Verification items for the finished model (mm, model axes). A direction names the side the tool comes from. Give positions to 0.01 mm unless a question says otherwise; leave off trailing zeros. Order: outer loops, then holes, each group sorted by start corner. A loop starts at its lowest first (then second) coordinate and runs counter-clockwise, first axis right, second up.
from build123d import *

# Parameters (mm, degrees)
BOSS_EXTRUDE2_DEPTH = 22
SHELL1_START        = -22
SHELL1_DEPTH        = 20
SKETCH2_W           = 99.356893422
SKETCH2_H           = 33.700277524
CUT_EXTRUDE1_DEPTH  = 20
SKETCH3_W           = 10.526500884
SKETCH3_H           = 10.645693642
CUT_EXTRUDE2_DEPTH  = 2
CUT_EXTRUDE3_DEPTH  = 2


# Read off the part's stored shape, not the designer's step: Shell1
with BuildPart() as part:
    # Sketch1 → Boss-Extrude2 (new body)
    with BuildSketch(Plane(origin=(0, 0, 0), x_dir=(1, 0, 0), z_dir=(0, 1, 0))):
        with BuildLine():
            Line((-51, 24.05), (51, 24.05))
            ThreePointArc((51, 24.05), (53.121320344, 23.171320344), (54, 21.05))
            Line((54, 21.05), (54, -16.2))
            ThreePointArc((54, -16.2), (53.121320344, -18.321320344), (51, -19.2))
            Line((51, -19.2), (-51, -19.2))
            ThreePointArc((-51, -19.2), (-53.121320344, -18.321320344), (-54, -16.2))
            Line((-54, -16.2), (-54, 21.05))
            ThreePointArc((-54, 21.05), (-53.121320344, 23.171320344), (-51, 24.05))
        make_face()
        with BuildLine():
            Line((-34.075, 9.25), (34.075, 9.25))
            ThreePointArc((34.075, 9.25), (43.325, 0), (34.075, -9.25))
            Line((34.075, -9.25), (-34.075, -9.25))
            ThreePointArc((-34.075, -9.25), (-43.325, 0), (-34.075, 9.25))
        make_face(mode=Mode.SUBTRACT)
    extrude(amount=-BOSS_EXTRUDE2_DEPTH)

    # Shell1 outline → Shell1 (cut)
    with BuildSketch(Plane(origin=(0, 0, 0), x_dir=(1, 0, 0), z_dir=(0, 1, 0)).offset(SHELL1_START)):
        with BuildLine():
            Line((-52, 21.05), (-52, -16.2))
            ThreePointArc((-52, -16.2), (-51.707106781, -16.907106781), (-51, -17.2))
            Line((-51, -17.2), (51, -17.2))
            ThreePointArc((51, -17.2), (51.707106781, -16.907106781), (52, -16.2))
            Line((52, -16.2), (52, 21.05))
            ThreePointArc((52, 21.05), (51.707106781, 21.757106781), (51, 22.05))
            Line((51, 22.05), (-51, 22.05))
            ThreePointArc((-51, 22.05), (-51.707106781, 21.757106781), (-52, 21.05))
        make_face()
        with BuildLine():
            ThreePointArc((-34.075, -11.25), (-45.325, 0), (-34.075, 11.25))
            Line((-34.075, 11.25), (34.075, 11.25))
            ThreePointArc((34.075, 11.25), (45.325, 0), (34.075, -11.25))
            Line((34.075, -11.25), (-34.075, -11.25))
        make_face(mode=Mode.SUBTRACT)
    extrude(amount=SHELL1_DEPTH, mode=Mode.SUBTRACT)

    # Sketch2 → Cut-Extrude1 (cut)
    with BuildSketch(Plane.XZ.offset(22)):
        Rectangle(SKETCH2_W, SKETCH2_H)
    extrude(amount=-CUT_EXTRUDE1_DEPTH, mode=Mode.SUBTRACT)

    # Sketch3 → Cut-Extrude2 (cut)
    with BuildSketch(Plane(origin=(0, 0, -24.05), x_dir=(-1, 0, 0), z_dir=(0, 0, -1))):
        with Locations((-43.321442995, -16.677153179)):
            Rectangle(SKETCH3_W, SKETCH3_H)
    extrude(amount=-CUT_EXTRUDE2_DEPTH, mode=Mode.SUBTRACT)

    # Sketch6 → Cut-Extrude3 (cut)
    with BuildSketch(Plane(origin=(0, 0, -24.05), x_dir=(-1, 0, 0), z_dir=(0, 0, -1))):
        with BuildLine():
            Line((46.497989358, -4.136848822), (-46.502010642, -4.136848822))
            ThreePointArc((-46.502010642, -4.136848822), (-47.502010642, -3.136848822), (-46.502010642, -2.136848822))
            Line((-46.502010642, -2.136848822), (46.497989358, -2.136848822))
            ThreePointArc((46.497989358, -2.136848822), (47.497989358, -3.136848822), (46.497989358, -4.136848822))
        make_face()
        with BuildLine():
            Line((46.497989358, -8.136848822), (-46.502010642, -8.136848822))
            ThreePointArc((-46.502010642, -8.136848822), (-47.502010642, -7.136848822), (-46.502010642, -6.136848822))
            Line((-46.502010642, -6.136848822), (46.497989358, -6.136848822))
            ThreePointArc((46.497989358, -6.136848822), (47.497989358, -7.136848822), (46.497989358, -8.136848822))
        make_face()
        with BuildLine():
            Line((-32.921100396, -9.626506099), (46.497989358, -9.626506099))
            ThreePointArc((46.497989358, -9.626506099), (47.497989358, -10.626506099), (46.497989358, -11.626506099))
            Line((46.497989358, -11.626506099), (-32.921100396, -11.626506099))
            ThreePointArc((-32.921100396, -11.626506099), (-33.921100396, -10.626506099), (-32.921100396, -9.626506099))
        make_face()
        with BuildLine():
            Line((-32.921100396, -13.626506099), (46.497989358, -13.626506099))
            ThreePointArc((46.497989358, -13.626506099), (47.497989358, -14.626506099), (46.497989358, -15.626506099))
            Line((46.497989358, -15.626506099), (-32.921100396, -15.626506099))
            ThreePointArc((-32.921100396, -15.626506099), (-33.921100396, -14.626506099), (-32.921100396, -13.626506099))
        make_face()
    extrude(amount=-CUT_EXTRUDE3_DEPTH, mode=Mode.SUBTRACT)


solid = part.part
(1) Go/stop test with flat-tipped pins: pin 1 (1.6 mm diameter, centred on y = -17, z = -23.5, fed in from -X); pin 2 (1 mm diameter, centred on y = -14.5, z = -23, fed in from +X); pin 3 (12 mm diameter, centred on x = 22, z = -11, fed in from -Y). Record where each tip stops, or that it passes through.
Solved:
pin 1: stops at x = -53.51
pin 2: stops at x = 53.63
pin 3: stops at y = -2
(2) Section check D-D, the plane z = -20. Enter the section's corners in (x, y), then the cut area to 3 significant figures.
Solved:
outline: (-54, -22) - (-52, -22) - (-52, -2) - (52, -2) - (52, -22) - (54, -22) - (54, 0) - (-54, 0) - close
area: 296 mm2
(3) Section check C-C, the plane y = -18.5. Enter the section's corners in (x, z).
Solved:
outline: (-54, -21.05) arc R3 ccw to (-51, -24.05) - (38.06, -24.05) - (38.06, -22.05) - (-51, -22.05) arc R1 cw to (-52, -21.05) - (-52, 16.2) arc R1 cw to (-51, 17.2) - (51, 17.2) arc R1 cw to (52, 16.2) - (52, -21.05) arc R1 cw to (51, -22.05) - (48.58, -22.05) - (48.58, -24.05) - (51, -24.05) arc R3 ccw to (54, -21.05) - (54, 16.2) arc R3 ccw to (51, 19.2) - (-51, 19.2) arc R3 ccw to (-54, 16.2) - close
(4) Release check for a two-part mould opening along Z. For faces 1 (the cylindrical face through (-43.323, -0.986, 0.203)), 2 (the flat face through (0, -1, 9.25)), 3 (the flat face through (1, -11, 19.2)), 4 (the flat face through (-1, -8.137, -23)) record: pulls with the +Z half, pulls with the -Z half, needs draft (parallel to the pull), parting line crosses it, or undercut.
Solved:
face 1: undercut
face 2: undercut
face 3: pulls with the +Z half
face 4: needs draft
(5) Set-up check for faces 5 (the flat face through (-1, -4.137, -23)), 6 (the flat face through (38.058, -17, -23)), 7 (the flat face through (-1, -12, 17.2)), 8 (the flat face through (0, -1, -9.25)): record each of +Z, -Z, +X, -X, +Y, -Y from which the full face is reachable in a straight line by a thin tool's end or side.
Solved:
face 5: -Z
face 6: -Z, -Y
face 7: -Y
face 8: +Y, -Y
(6) Section check B-B, the plane z = 0. Enter the section's corners in (x, y) (3 decimals), then the cut area to 3 significant figures.
Solved:
outline: (-54, -22) - (-52, -22) - (-52, -2) - (-43.325, -2) - (-43.325, 0) - (-54, 0) - close; (43.325, -2) - (52, -2) - (52, -22) - (54, -22) - (54, 0) - (43.325, 0) - close
area: 123 mm2
(7) Scan lines: line 1 (Z direction, x = 37, y = -18.5); line 2 (X direction, y = -8, z = -15.5). Record each from-to range of solid material in increasing order.
Solved:
line 1: z = -24.05 to -22.05, 17.2 to 19.2
line 2: x = -54 to -52, 52 to 54
(8) Section check A-A, the plane x = -16. Enter the section's corners in (y, z), then the cut area to 4 significant figures.
Solved:
outline: (-22, -24.05) - (-15.63, -24.05) - (-15.63, -22.05) - (-22, -22.05) - close; (-22, 17.2) - (-2, 17.2) - (-2, 9.25) - (0, 9.25) - (0, 19.2) - (-22, 19.2) - close; (-13.63, -24.05) - (-11.63, -24.05) - (-11.63, -22.05) - (-13.63, -22.05) - close; (-9.63, -24.05) - (-8.14, -24.05) - (-8.14, -22.05) - (-9.63, -22.05) - close; (-6.14, -24.05) - (-4.14, -24.05) - (-4.14, -22.05) - (-6.14, -22.05) - close; (-2.14, -24.05) - (0, -24.05) - (0, -9.25) - (-2, -9.25) - (-2, -22.05) - (-2.14, -22.05) - close
area: 113.5 mm2
